```python
from build123d import *

# Parameters (mm, degrees)
SKETCH_1_W           = 290
SKETCH_1_H           = 190
EXTRUDE_1_DEPTH      = 2
SKETCH_2_W           = 22
SKETCH_2_H           = 22
CUT_EXTRUDE_1_DEPTH  = 2
FILLET_2_R           = 3
FILLET_3_R           = 3
SKETCH_3_W           = 50
SKETCH_3_H           = 30
CUT_EXTRUDE_2_DEPTH  = 10
FILLET_4_R           = 3
CUT_EXTRUDE_3_DEPTH  = 10
FILLET_5_R           = 3
SKETCH_5_R           = 1.75
SKETCH_5_R_2         = 1.5
CUT_EXTRUDE_4_DEPTH  = 10
SKETCH_6_W           = 38.367930324
SKETCH_6_H           = 26
SKETCH_6_W_2         = 43.939038981
CUT_EXTRUDE_5_DEPTH  = 10
FILLET_6_R           = 3
SKETCH_7_R           = 1.75
CUT_EXTRUDE_6_DEPTH  = 10
SKETCH_8_W           = 43
SKETCH_8_H           = 46
CUT_EXTRUDE_7_DEPTH  = 10
FILLET_7_R           = 3
SKETCH_10_R          = 11
SKETCH_10_W          = 40
SKETCH_10_H          = 42
SKETCH_10_W_2        = 36
SKETCH_10_H_2        = 30
CUT_EXTRUDE_9_DEPTH  = 10
SKETCH_11_R          = 1.75
CUT_EXTRUDE_10_DEPTH = 10
SKETCH_9_W           = 50
SKETCH_9_H           = 55
CUT_EXTRUDE_11_DEPTH = 10
FILLET_8_R           = 3


with BuildPart() as part:
    # 草图1 → 凸台-拉伸1 (new body)
    with BuildSketch(Plane.XY):
        Rectangle(SKETCH_1_W, SKETCH_1_H)
    extrude(amount=EXTRUDE_1_DEPTH)

    # 草图2 → 切除-拉伸1 (cut)
    with BuildSketch(Plane(origin=(0, 0, 0), x_dir=(-1, 0, 0), z_dir=(0, 0, -1))):
        with Locations((-134, 84)):
            Rectangle(SKETCH_2_W, SKETCH_2_H)
        with Locations((134, 84)):
            Rectangle(SKETCH_2_W, SKETCH_2_H)
        Polygon((-125, -72), (-145, -72), (-145, -111.869716796), (-117, -111.869716796), (-117, -72), align=None)
        Polygon((117, -72), (125, -72), (145, -72), (145, -111.869716796), (117, -111.869716796), align=None)
    extrude(amount=-CUT_EXTRUDE_1_DEPTH, mode=Mode.SUBTRACT)

    # 圆角2
    fillet_2_edges = [part.edges().sort_by_distance(p)[0] for p in [
        (117, -72, 1),
        (-117, -72, 1),
    ]]
    fillet(fillet_2_edges, radius=FILLET_2_R)

    # 圆角3
    fillet_3_edges = [part.edges().sort_by_distance(p)[0] for p in [
        (-123, 73, 1),
        (123, 73, 1),
    ]]
    fillet(fillet_3_edges, radius=FILLET_3_R)

    # 草图3 → 切除-拉伸2 (cut)
    with BuildSketch(Plane.XY.offset(2)):
        with Locations((0, 80)):
            Rectangle(SKETCH_3_W, SKETCH_3_H)
    extrude(amount=-CUT_EXTRUDE_2_DEPTH, mode=Mode.SUBTRACT)

    # 圆角4
    fillet_4_edges = [part.edges().sort_by_distance(p)[0] for p in [
        (25, 65, 1),
        (-25, 65, 1),
    ]]
    fillet(fillet_4_edges, radius=FILLET_4_R)

    # 草图4 → 切除-拉伸3 (cut)
    with BuildSketch(Plane(origin=(0, 0, 0), x_dir=(-1, 0, 0), z_dir=(0, 0, -1))):
        Polygon((18.975534939, -95.441726104), (29.469060061, -1), (-29.469060061, -1), (-18.975534939, -95.441726104), align=None)
    extrude(amount=-CUT_EXTRUDE_3_DEPTH, mode=Mode.SUBTRACT)

    # 圆角5
    fillet_5_edges = [part.edges().sort_by_distance(p)[0] for p in [
        (29.469060061, -1, 1),
        (-29.469060061, -1, 1),
    ]]
    fillet(fillet_5_edges, radius=FILLET_5_R)

    # 草图5 → 切除-拉伸4 (cut)
    with BuildSketch(Plane(origin=(0, 0, 0), x_dir=(-1, 0, 0), z_dir=(0, 0, -1))):
        with Locations((65, -85)):
            Circle(SKETCH_5_R)
        with Locations((105, -85)):
            Circle(SKETCH_5_R_2)
        with Locations((135, -35)):
            Circle(SKETCH_5_R_2)
        with Locations((-65, -85)):
            Circle(SKETCH_5_R)
        with Locations((-135, -65)):
            Circle(SKETCH_5_R_2)
        with Locations((-135, -35)):
            Circle(SKETCH_5_R_2)
        with Locations((-135, 45)):
            Circle(SKETCH_5_R_2)
        with Locations((-135, 65)):
            Circle(SKETCH_5_R_2)
        with Locations((-115, 85)):
            Circle(SKETCH_5_R_2)
        with Locations((-95, 85)):
            Circle(SKETCH_5_R_2)
        with Locations((95, 85)):
            Circle(SKETCH_5_R_2)
        with Locations((115, 85)):
            Circle(SKETCH_5_R_2)
        with Locations((135, 65)):
            Circle(SKETCH_5_R_2)
        with Locations((135, 45)):
            Circle(SKETCH_5_R_2)
        with Locations((135, -65)):
            Circle(SKETCH_5_R_2)
        with Locations((-105, -85)):
            Circle(SKETCH_5_R_2)
    extrude(amount=-CUT_EXTRUDE_4_DEPTH, mode=Mode.SUBTRACT)

    # 草图6 → 切除-拉伸5 (cut)
    with BuildSketch(Plane(origin=(0, 0, 0), x_dir=(-1, 0, 0), z_dir=(0, 0, -1))):
        with Locations((136.183965162, -15)):
            Rectangle(SKETCH_6_W, SKETCH_6_H)
        with Locations((-138.969519491, -15)):
            Rectangle(SKETCH_6_W_2, SKETCH_6_H)
    extrude(amount=-CUT_EXTRUDE_5_DEPTH, mode=Mode.SUBTRACT)

    # 圆角6
    fillet_6_edges = [part.edges().sort_by_distance(p)[0] for p in [
        (117, -2, 1),
        (117, -28, 1),
        (-117, -28, 1),
        (-117, -2, 1),
    ]]
    fillet(fillet_6_edges, radius=FILLET_6_R)

    # 草图7 → 切除-拉伸6 (cut)
    with BuildSketch(Plane(origin=(0, 0, 0), x_dir=(-1, 0, 0), z_dir=(0, 0, -1))):
        with Locations((81.75, -70)):
            Circle(SKETCH_7_R)
        with Locations((32.75, -70)):
            Circle(SKETCH_7_R)
        with Locations((32.75, -30)):
            Circle(SKETCH_7_R)
        with Locations((81.75, -30)):
            Circle(SKETCH_7_R)
        with Locations((-81.75, -70)):
            Circle(SKETCH_7_R)
        with Locations((-32.75, -70)):
            Circle(SKETCH_7_R)
        with Locations((-32.75, -30)):
            Circle(SKETCH_7_R)
        with Locations((-81.75, -30)):
            Circle(SKETCH_7_R)
        with Locations((-120, 30)):
            Circle(SKETCH_7_R)
        with Locations((-120, 70)):
            Circle(SKETCH_7_R)
        with Locations((-71, 70)):
            Circle(SKETCH_7_R)
        with Locations((-71, 30)):
            Circle(SKETCH_7_R)
        with Locations((71, 70)):
            Circle(SKETCH_7_R)
        with Locations((120, 30)):
            Circle(SKETCH_7_R)
        with Locations((71, 30)):
            Circle(SKETCH_7_R)
        with Locations((120, 70)):
            Circle(SKETCH_7_R)
    extrude(amount=-CUT_EXTRUDE_6_DEPTH, mode=Mode.SUBTRACT)

    # 草图8 → 切除-拉伸7 (cut)
    with BuildSketch(Plane(origin=(0, 0, 0), x_dir=(-1, 0, 0), z_dir=(0, 0, -1))):
        with Locations((-95.5, 50)):
            Rectangle(SKETCH_8_W, SKETCH_8_H)
        with Locations((-57.25, -50)):
            Rectangle(SKETCH_8_W, SKETCH_8_H)
        with Locations((57.25, -50)):
            Rectangle(SKETCH_8_W, SKETCH_8_H)
        with Locations((95.5, 50)):
            Rectangle(SKETCH_8_W, SKETCH_8_H)
    extrude(amount=-CUT_EXTRUDE_7_DEPTH, mode=Mode.SUBTRACT)

    # 圆角7
    fillet_7_edges = [part.edges().sort_by_distance(p)[0] for p in [
        (-117, 73, 1),
        (-117, 27, 1),
        (-74, 27, 1),
        (-74, 73, 1),
        (-78.75, -27, 1),
        (-78.75, -73, 1),
        (-35.75, -73, 1),
        (-35.75, -27, 1),
        (35.75, -27, 1),
        (35.75, -73, 1),
        (78.75, -73, 1),
        (78.75, -27, 1),
        (74, 73, 1),
        (74, 27, 1),
        (117, 27, 1),
        (117, 73, 1),
    ]]
    fillet(fillet_7_edges, radius=FILLET_7_R)

    # 草图10 → 切除-拉伸9 (cut)
    with BuildSketch(Plane.XY.offset(2)):
        with Locations((-46.436017542, 77.667392483)):
            Circle(SKETCH_10_R)
        with Locations(Location((46.436017542, 77.667392483, 0), (0, 0, 180))):
            Circle(SKETCH_10_R)
        with Locations((91.396155993, 0)):
            Rectangle(SKETCH_10_W, SKETCH_10_H)
        with Locations((-91.396155993, 0)):
            Rectangle(SKETCH_10_W, SKETCH_10_H)
        with Locations((-109.352757312, -50.443602375)):
            Rectangle(SKETCH_10_W_2, SKETCH_10_H_2)
        with Locations((109.352757312, -50.443602375)):
            Rectangle(SKETCH_10_W_2, SKETCH_10_H_2)
    extrude(amount=-CUT_EXTRUDE_9_DEPTH, mode=Mode.SUBTRACT)

    # 草图11 → 切除-拉伸10 (cut)
    with BuildSketch(Plane(origin=(0, 0, 0), x_dir=(-1, 0, 0), z_dir=(0, 0, -1))):
        with Locations((7.5, 10.5)):
            Circle(SKETCH_11_R)
        with Locations((-7.5, 10.5)):
            Circle(SKETCH_11_R)
        with Locations((7.5, 28.5)):
            Circle(SKETCH_11_R)
        with Locations((-7.5, 28.5)):
            Circle(SKETCH_11_R)
    extrude(amount=-CUT_EXTRUDE_10_DEPTH, mode=Mode.SUBTRACT)

    # 草图9 → 切除-拉伸11 (cut)
    with BuildSketch(Plane(origin=(0, 0, 0), x_dir=(-1, 0, 0), z_dir=(0, 0, -1))):
        with Locations((-39, 32)):
            Rectangle(SKETCH_9_W, SKETCH_9_H)
        with Locations((39, 32)):
            Rectangle(SKETCH_9_W, SKETCH_9_H)
    extrude(amount=-CUT_EXTRUDE_11_DEPTH, mode=Mode.SUBTRACT)

    # 圆角8
    fillet_8_edges = [part.edges().sort_by_distance(p)[0] for p in [
        (14, 59.5, 1),
        (14, 4.5, 1),
        (64, 4.5, 1),
        (64, 59.5, 1),
        (-64, 59.5, 1),
        (-64, 4.5, 1),
        (-14, 4.5, 1),
        (-14, 59.5, 1),
    ]]
    fillet(fillet_8_edges, radius=FILLET_8_R)


solid = part.part
```
Source: CAD feature listing. Evaluate the final solid. Frame: model axes, mm. A direction names the side the tool comes from. Coordinates: 2 decimals unless noted, no trailing zeros. Answer as a JSON object with one key per item and string values.
1. Access query for faces 3 (the flat face through (-23.99, -50.3, 0.99)), 4 (the flat face through (-2, 1, 2)). Directions: +Z, -Z, +X, -X, +Y, -Y. A direction counts if a zero-diameter tool reaches every point of the face in a straight line with its end or side. Return the directions, or none.
Evaluation:
{"face 3": "+Z, -Z", "face 4": "+Z, +X, -X, +Y, -Y"}
2. Cut plane A-A on z = 0.6. State how many separate pieces and enclosed holes the cut face has, plus the area to 3 significant figures.
Evaluation:
{"separate pieces": "1", "enclosed holes": "48", "area": "25,400 mm^2"}
3. Contact query for a flat-ended pin moving along its axis: P1, Ø1, axis at x = 136, z = 1, coming from the +Y side. Output: stop coordinate, or through.
Evaluation:
{"P1": "y = 73"}
4. Ray query, L1, parallel to Y at x = 81.75, z = 0.85; L2, parallel to X at y = 55, z = 0.35; L3, parallel to Y at x = -109, z = 1.2. Return the intervals inside material, ascending.
Evaluation:
{"L1": "-95 to -71.75, -68.25 to -31.75, -28.25 to -21, 21 to 27, 73 to 95", "L2": "-145 to -117, -74 to -64, -14 to 14, 64 to 74, 117 to 145", "L3": "-95 to -65.44, -35.44 to -21, 21 to 27, 73 to 95"}
5. Draft query along X for faces 1 (the flat face through (-2, 1, 0)), 2 (the cylindrical face through (55.165, 84.361, 1.014)). Return one class per face: released by +X, released by -X, zero draft, split by the parting line, or undercut.
Evaluation:
{"face 1": "zero draft", "face 2": "undercut"}
